from build123d import *

# Parameters (mm, degrees)
SKETCH1_W             = 145
SKETCH1_H             = 145
BOSS_EXTRUDE179_DEPTH = 3
SKETCH2_W             = 40
SKETCH2_H             = 3
SKETCH2_W_2           = 3
SKETCH2_H_2           = 40
CUT_EXTRUDE1_DEPTH    = 3


with BuildPart() as part:
    # Sketch1 → Boss-Extrude179 (new body)
    with BuildSketch(Plane.XY):
        Rectangle(SKETCH1_W, SKETCH1_H)
    extrude(amount=BOSS_EXTRUDE179_DEPTH)

    # Sketch2 → Cut-Extrude1 (cut)
    with BuildSketch(Plane.XY.offset(3)):
        with Locations((-32.5, 71)):
            Rectangle(SKETCH2_W, SKETCH2_H)
        with Locations((32.5, 71)):
            Rectangle(SKETCH2_W, SKETCH2_H)
        with Locations((-71, 32.5)):
            Rectangle(SKETCH2_W_2, SKETCH2_H_2)
        with Locations((-71, -32.5)):
            Rectangle(SKETCH2_W_2, SKETCH2_H_2)
        with Locations((32.5, -71)):
            Rectangle(SKETCH2_W, SKETCH2_H)
        with Locations((-32.5, -71)):
            Rectangle(SKETCH2_W, SKETCH2_H)
        with Locations((71, -32.5)):
            Rectangle(SKETCH2_W_2, SKETCH2_H_2)
        with Locations((71, 32.5)):
            Rectangle(SKETCH2_W_2, SKETCH2_H_2)
    extrude(amount=-CUT_EXTRUDE1_DEPTH, mode=Mode.SUBTRACT)


solid = part.part
Geometry check sheet. Reference: the model listing, model coordinates, mm. Coordinates: 2 decimals unless noted, no trailing zeros. Order: outer loops, then holes, each group sorted by start corner. A loop starts at its lowest first (then second) coordinate and runs counter-clockwise, first axis right, second up. Notation, with made-up numbers: (38, -22) -> (53, -22) arc R26 ccw to (53, -3) -> close; hole circle Ø5 at (14.5, 60). An arc over 180 degrees is marked (long way). Use a Markdown table: item, result. Add a question column.
1. Go/stop test with flat-tipped pins: pin 1 Ø0.9 at (x, z) = (-39, 1.5) entering from +Y; pin 2 Ø0.9 at (x, z) = (38, 1) entering from -Y. Record where each tip stops, or that it passes through.
2. Cross-section at A-A (x = 50). Enter the section's corners in (y, z).
3. Material ranges on L1, parallel to Y at x = -35.5, z = 2.65, recorded low to high.
Filled sheet:
| question | item | result |
|---|---|---|
| 1 | pin 1 | y = 69.5 |
| 1 | pin 2 | y = -69.5 |
| 2 | outline | (-69.5, 0) -> (69.5, 0) -> (69.5, 3) -> (-69.5, 3) -> close |
| 3 | L1 | -69.5 to 69.5 |
